Can you work these out from the drawing? Everything is in mm from the part's minimum corner. Round coordinates to 2 decimals unless told otherwise and drop trailing zeros. Write each loop counter-clockwise with the first axis right and the second up, starting at its lowest first coordinate (ties: lowest second). Pieces come first, ordered by that corner, then holes. Notation, with made-up numbers: (18.25, 82.5) - (39.25, 82.5) arc R32 ccw to (39.25, 111.5) - close; hole circle Ø11 at (11.25, 16). An arc over 180 degrees is marked (long way). Write each question's results on one line, items separated by ' | '. Start each with the question number.
(1) For P1, Ø1, axis at x = 16.5, y = 28, coming from the +Z side, with a flat end and sliding along its axis, tell me the tip position at first contact or that it passes through.
(2) Please list where these lines run through material, in increasing order: line 1 (Y direction, x = 14, z = 4.25); line 2 (Z direction, x = 8, y = 5.75); line 3 (Y direction, x = 12, z = 5). Write a range as [from, to].
(3) Imagine slicing it at B-B on y = 28. Write out the boundary of the cut face in (x, z), then the cut area to 3 significant figures.
(4) Imagine slicing it at A-A on y = 10. Write out the boundary of the cut face in (x, z).
(5) Thinking about a two-plate mould opening in Y: for the marked faces 1, 2 and 3, which applies, +Y half, -Y half, draft (parallel to the pull), parting line (faces both ways), or undercut?
(6) Imagine slicing it at D-D on z = 7.5. Write out the boundary of the cut face in (x, y), then the cut area to 3 significant figures.
(7) Imagine slicing it at C-C on x = 14. Write out the boundary of the cut face in (y, z), then the cut area to 3 significant figures.
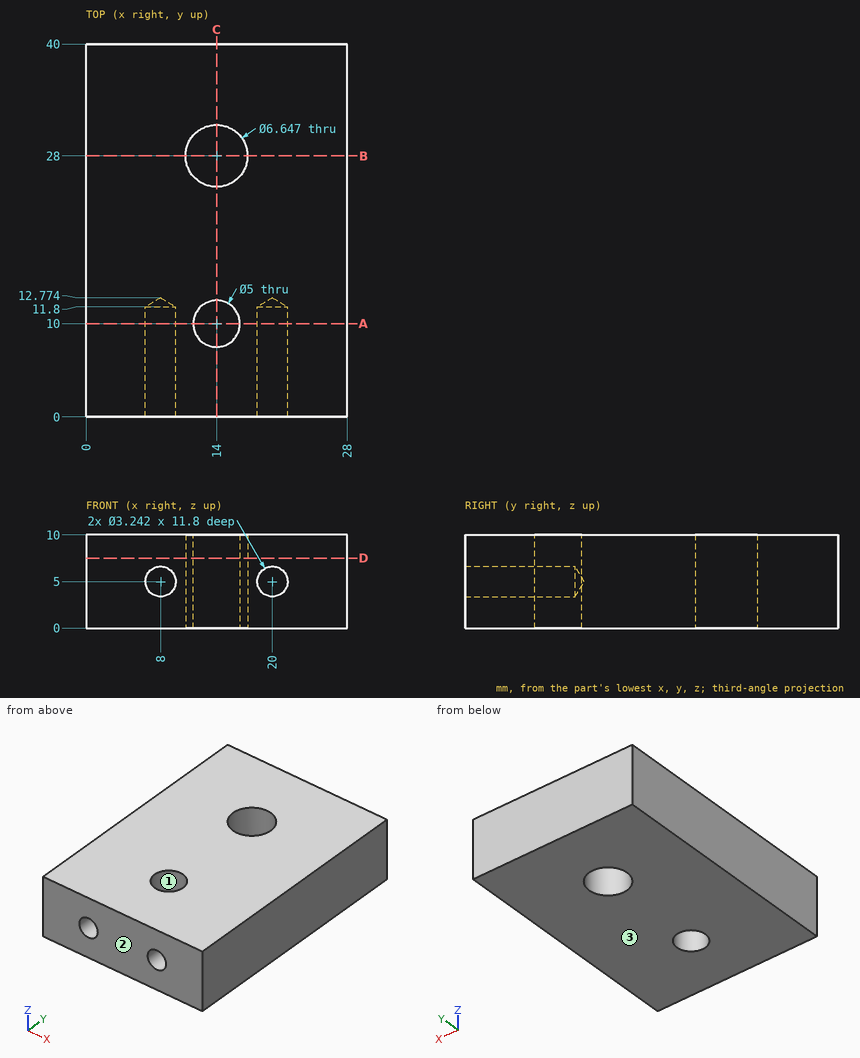
Response:
1) P1: through
2) line 1: [0, 7.5], [12.5, 24.68], [31.32, 40] | line 2: [0, 3.38], [6.62, 10] | line 3: [0, 8.5], [11.5, 25.35], [30.65, 40]
3) outline: (0, 0) - (10.68, 0) - (10.68, 10) - (0, 10) - close; (17.32, 0) - (28, 0) - (28, 10) - (17.32, 10) - close | area: 214 mm²
4) outline: (0, 0) - (11.5, 0) - (11.5, 10) - (0, 10) - close; (16.5, 0) - (28, 0) - (28, 10) - (16.5, 10) - close; hole circle Ø3.24 at (8, 5); hole circle Ø3.24 at (20, 5)
5) face 1: undercut | face 2: -Y half | face 3: draft
6) outline: (0, 0) - (28, 0) - (28, 40) - (0, 40) - close; hole circle Ø6.65 at (14, 28); hole circle Ø5 at (14, 10) | area: 1,070 mm²
7) outline: (0, 0) - (7.5, 0) - (7.5, 10) - (0, 10) - close; (12.5, 0) - (24.68, 0) - (24.68, 10) - (12.5, 10) - close; (31.32, 0) - (40, 0) - (40, 10) - (31.32, 10) - close | area: 284 mm²
